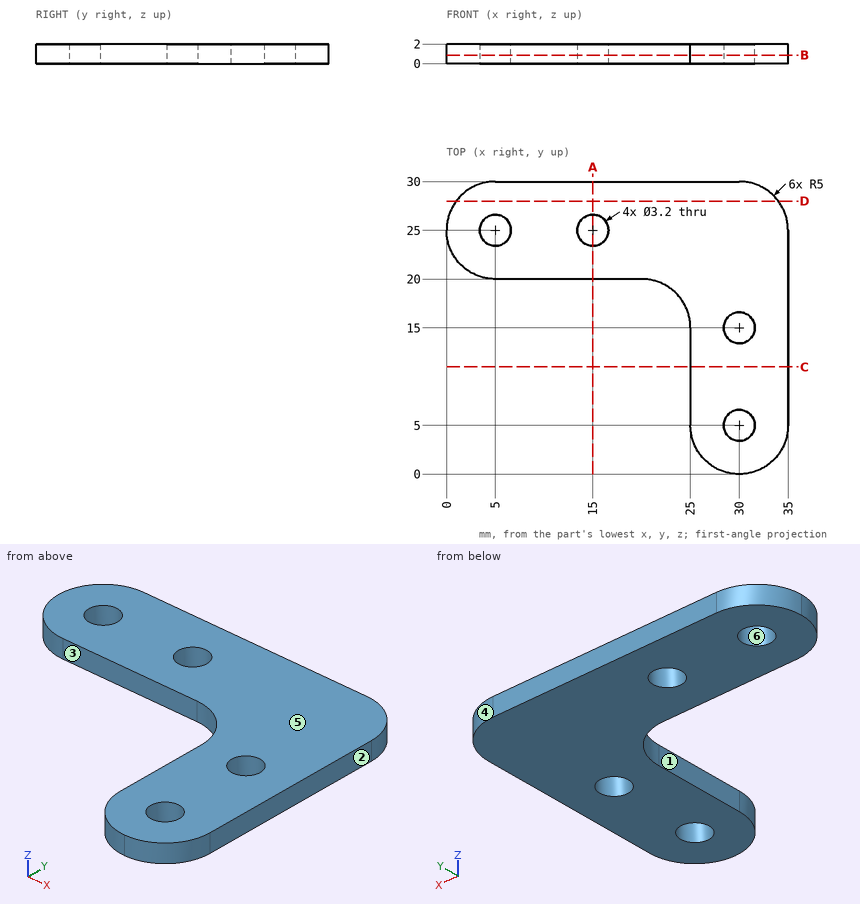
Source: three-view drawing plus pictorial views. Frame: mm from the lowest corner of the part. A direction names the side the tool comes from. Round coordinates to 2 decimals unless told otherwise and drop trailing zeros. Order: outer loops, then holes, each group sorted by start corner. A loop starts at its lowest first (then second) coordinate and runs counter-clockwise, first axis right, second up. Notation, with made-up numbers: (59.25, -5.5) -> (116.25, -5.5) arc R17 ccw to (116.25, 26.5) -> close; hole circle Ø10 at (10.25, 79). An arc over 180 degrees is marked (long way). Use one line per item in the form item = value. Start each with the question number.
1. Cut plane B-B (z = 0.85). Count the separate pieces of the cut face and the enclosed holes in it, then the cut area to 3 significant figures.
2. Line query: probe 1 along Y at (x, z) = (30, 1.05); probe 2 along X at (y, z) = (5, 0.5); probe 3 along Y at (x, z) = (15, 0.1). Output: solid intervals per line, ascending.
3. Reachability of the marked faces 1 and 2 from +Z, -Z, +X, -X, +Y, -Y: full face, straight path, thin tool, end or side. Return the list, or none.
4. Cut plane C-C (y = 11). Return the cut outline in (x, z).
5. Pin query (flat end, axial travel): pin 1 Ø0.6 at (x, z) = (12.5, 0.5) entering from -Y; pin 2 Ø2.5 at (x, y) = (30, 5) entering from -Z. Return the tip coordinate at first contact, or that it passes through.
6. Cut plane A-A (x = 15). Return the cut outline in (y, z), then the cut area to 3 significant figures.
7. Draft query along Y for the marked faces 3, 4, 5 and 6. Return one class per face: pulls with the +Y half, pulls with the -Y half, needs draft (parallel to the pull), parting line crosses it, or undercut.
8. Cut plane D-D (y = 28). Return the cut outline in (x, z), then the cut area to 3 significant figures.
Solution:
q1.separate_pieces = 1
q1.enclosed_holes = 4
q1.area = 496 mm^2
q2.probe_1 = 0 to 3.4, 6.6 to 13.4, 16.6 to 30
q2.probe_2 = 25 to 28.4, 31.6 to 35
q2.probe_3 = 20 to 23.4, 26.6 to 30
q3.face_1 = +Z, -Z, -X, -Y
q3.face_2 = +Z, -Z, +X, +Y, -Y
q4.outline = (25, 0) -> (35, 0) -> (35, 2) -> (25, 2) -> close
q5.pin_1 = 20
q5.pin_2 = through
q6.outline = (20, 0) -> (23.4, 0) -> (23.4, 2) -> (20, 2) -> close; (26.6, 0) -> (30, 0) -> (30, 2) -> (26.6, 2) -> close
q6.area = 13.6 mm^2
q7.face_3 = pulls with the -Y half
q7.face_4 = pulls with the +Y half
q7.face_5 = needs draft
q7.face_6 = undercut
q8.outline = (1, 0) -> (34, 0) -> (34, 2) -> (1, 2) -> close
q8.area = 66.0 mm^2
